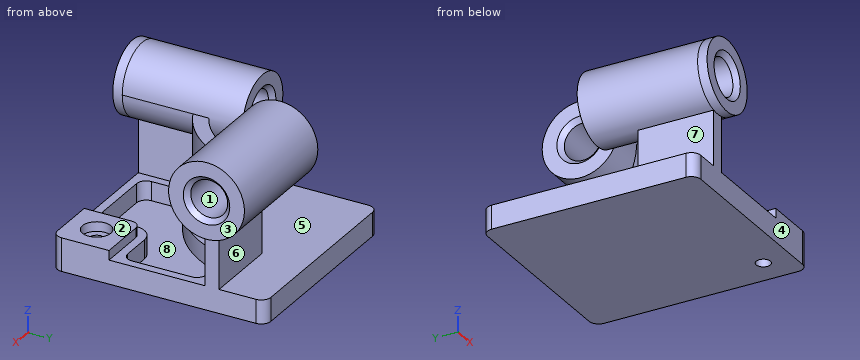
from build123d import *

# Parameters (mm, degrees)
F0_W            = 210
F0_H            = 225
F1_DEPTH        = 25
F3_DEPTH        = 95
F4_R            = 37.5
F5_DEPTH        = 10
F5_DEPTH_BACK   = 127
F6_R            = 40
F7_DEPTH        = 10
F7_DEPTH_BACK   = 127
F8_W            = 60
F8_H            = 60
F9_DEPTH        = 10
F10_R           = 10
F12_DEPTH       = 20
F14_D           = 15
F14_CBORE_D     = 30
F14_CBORE_DEPTH = 10
F15_R           = 10
F16_R           = 19.5
F17_DEPTH       = 235.001
F18_R           = 19.5
F19_DEPTH       = 220.001
F20_SIZE        = 5
F21_R           = 10


with BuildPart() as f1:
    # F0 (on Top) → F1 (new body)
    with BuildSketch(Plane.XY):
        Rectangle(F0_W, F0_H)
    extrude(amount=F1_DEPTH)

    # F2 (on face) → F3 (join)
    with BuildSketch(Plane.XY.offset(25)):
        with BuildLine():
            Line((-71, -32.5), (-71, -112.5))
            Line((-71, -112.5), (-56, -112.5))
            Line((-56, -112.5), (-56, -46.481817))
            ThreePointArc((-56, -46.481817), (7.488853, -14.988853), (38.981817, 48.5))
            Line((38.981817, 48.5), (105, 48.5))
            Line((105, 48.5), (105, 63.5))
            Line((105, 63.5), (25, 63.5))
            ThreePointArc((25, 63.5), (-3.117749, -4.382251), (-71, -32.5))
        make_face()
    extrude(amount=F3_DEPTH)

    # F4 (on face) → F5 (join, two sides)
    with BuildSketch(Plane.XZ.offset(112.5)) as f5_sk:
        with Locations((-63.5, 120)):
            Circle(F4_R)
    extrude(amount=F5_DEPTH)
    extrude(f5_sk.sketch, amount=-F5_DEPTH_BACK)

    # F6 (on face) → F7 (join, two sides)
    with BuildSketch(Plane.YZ.offset(105)) as f7_sk:
        with Locations((56, 120)):
            Circle(F6_R)
    extrude(amount=F7_DEPTH)
    extrude(f7_sk.sketch, amount=-F7_DEPTH_BACK)

    # F8 (on face) → F9 (join)
    with BuildSketch(Plane.XY.offset(25)):
        with Locations((75, -82.5)):
            Rectangle(F8_W, F8_H)
    extrude(amount=F9_DEPTH)

    # F10
    f10_edges = [f1.edges().sort_by_distance(p)[0] for p in [
        (45, -52.5, 30),
    ]]
    fillet(f10_edges, radius=F10_R)

    # F11 (on face) → F12 (cut)
    with BuildSketch(Plane.XY.offset(25)):
        with BuildLine():
            ThreePointArc((46.575508, 39.5), (13.852814, -21.352814), (-47, -54.075508))
            Line((-47, -54.075508), (-47, -103.5))
            Line((-47, -103.5), (36, -103.5))
            Line((36, -103.5), (36, -62.5))
            ThreePointArc((36, -62.5), (41.564971, -49.064971), (55, -43.5))
            Line((55, -43.5), (96, -43.5))
            Line((96, -43.5), (96, 39.5))
            Line((96, 39.5), (46.575508, 39.5))
        make_face()
    extrude(amount=-F12_DEPTH, mode=Mode.SUBTRACT)

    # F14 (through all)
    with Locations(Plane.XY.offset(35)):
        with Locations((75, -82.5)):
            CounterBoreHole(F14_D / 2, F14_CBORE_D / 2, F14_CBORE_DEPTH)

    # F15
    f15_edges = [f1.edges().sort_by_distance(p)[0] for p in [
        (-47, -54.075508, 15),
        (46.575508, 39.5, 15),
        (96, 39.5, 15),
        (96, -43.5, 15),
        (36, -103.5, 15),
        (-47, -103.5, 15),
    ]]
    fillet(f15_edges, radius=F15_R)

    # F16 (on face) → F17 (cut, through all)
    with BuildSketch(Plane.XZ.offset(122.5)):
        with Locations((-63.5, 120)):
            Circle(F16_R)
    extrude(amount=-F17_DEPTH, mode=Mode.SUBTRACT)

    # F18 (on face) → F19 (cut, through all)
    with BuildSketch(Plane.YZ.offset(115)):
        with Locations((56, 120)):
            Circle(F18_R)
    extrude(amount=-F19_DEPTH, mode=Mode.SUBTRACT)

    # F20
    f20_edges = [f1.edges().sort_by_distance(p)[0] for p in [
        (115, 36.5, 120),
        (-22, 36.5, 120),
        (-83, 14.5, 120),
        (-83, -122.5, 120),
    ]]
    chamfer(f20_edges, length=F20_SIZE)

    # F21
    f21_edges = [f1.edges().sort_by_distance(p)[0] for p in [
        (-105, -112.5, 12.5),
        (105, -112.5, 17.5),
        (105, 112.5, 12.5),
        (-105, 112.5, 12.5),
    ]]
    fillet(f21_edges, radius=F21_R)


solid = f1.part
The listing builds one solid part. Answer for the finished solid, in the listing's coordinates (mm). Face numbers are marked on the shaded views. A direction names the side the tool comes from. Coordinates: 2 decimals unless noted, no trailing zeros. Write each loop counter-clockwise with the first axis right and the second up, starting at its lowest first coordinate (ties: lowest second). Pieces come first, ordered by that corner, then holes. Notation, with made-up numbers: M 49,52 L 91,52 A21 cw 91,72 Z; hole C 76,73 d10. An arc over 180 degrees is marked long. Put each result on its own line as item: value. Start each with the question number.
1. For a pull along Z with two mould halves and no side action, classify the marked faces 1, 2 and 3 as pulls with the +Z half, pulls with the -Z half, needs draft (parallel to the pull), parting line crosses it, or undercut.
2. A cutting plane is placed at B-B on x = 75. Write down the section's boundary in (y, z), then the cut area to 3 significant figures.
3. A cutting plane is placed at A-A on y = -82.5. Write down the section's boundary in (x, z), then the cut area to 3 significant figures.
4. Consider line 1 (Y direction, x = 75, z = 19); line 2 (Z direction, x = 42.5, y = 56); line 3 (Z direction, x = -75.5, y = 10.5). Determine where each line is inside the solid, lowest interval first. Write a range as from..to.
5. A cutting plane is placed at C-C on z = 17. Write down the section's boundary in (x, y), then the cut area to 3 significant figures.
6. Flat-ended cylindrical pins translate along their axes: P1, Ø9, axis at x = 75, y = -82.5, coming from the -Z side; P2, Ø18, axis at x = 67.5, y = -69, coming from the +Z side; P3, Ø25, axis at x = -9.5, z = 38.5, coming from the -Y side; P4, Ø16, axis at y = -72, z = 17, coming from the +X side. Find the tip coordinate at first contact, or state that the pin passes through.
7. Which of the six approach directions +Z, -Z, +X, -X, +Y, -Y give full straight-line access (tool end or side, diameter ignored) to the marked faces 4, 5, 6, 7 and 8?
8. A cutting plane is placed at D-D on x = 49. Write down the section's boundary in (y, z), then the cut area to 3 significant figures.
Resolved:
1. face 1: undercut
1. face 2: pulls with the +Z half
1. face 3: needs draft
2. outline: M -112.5,0 L -90,0 L -90,25 L -97.5,25 L -97.5,35 L -112.5,35 Z; M -75,0 L 112.5,0 L 112.5,25 L 63.5,25 L 63.5,80.71 A40 ccw long 48.5,80.71 L 48.5,25 L 39.5,25 L 39.5,5 L -43.5,5 L -43.5,25 L -52.5,25 L -52.5,35 L -67.5,35 L -67.5,25 L -75,25 Z; hole C 56,120 d39
2. area: 8,550 mm2
3. outline: M -105,0 L 67.5,0 L 67.5,25 L 60,25 L 60,35 L 45,35 L 45,25 L 36,25 L 36,5 L -47,5 L -47,25 L -56,25 L -56,83.26 A37.5 ccw long -71,83.26 L -71,25 L -105,25 Z; M 82.5,0 L 105,0 L 105,35 L 90,35 L 90,25 L 82.5,25 Z; hole C -63.5,120 d39
3. area: 7,600 mm2
4. line 1: y = -112.5..-90, -75..-43.5, 39.5..112.5
4. line 2: z = 0..100.5, 139.5..160
4. line 3: z = 0..25, 84.47..103.38, 136.62..155.53
5. outline: M -105,-102.5 A10 ccw -95,-112.5 L 95,-112.5 A10 ccw 105,-102.5 L 105,102.5 A10 ccw 95,112.5 L -95,112.5 A10 ccw -105,102.5 Z; hole M -47,-93.5 A10 ccw -37,-103.5 L 26,-103.5 A10 ccw 36,-93.5 L 36,-62.5 A19 cw 55,-43.5 L 86,-43.5 A10 ccw 96,-33.5 L 96,29.5 A10 ccw 86,39.5 L 54.48,39.5 A10 ccw 44.82,32.12 A120 cw -39.62,-52.32 A10 ccw -47,-61.98 Z; hole C 75,-82.5 d15
5. area: 36,300 mm2
6. P1: passes through
6. P2: stops at z = 35
6. P3: stops at y = -36.1
6. P4: stops at x = 105
7. face 4: -Z, +X, -X, -Y
7. face 5: -X, +Y
7. face 6: +X, -X, +Y
7. face 7: -X, +Y, -Y
7. face 8: none
8. outline: M -112.5,0 L 112.5,0 L 112.5,25 L 63.5,25 L 63.5,80.71 A40 ccw long 48.5,80.71 L 48.5,25 L 37.87,25 L 37.87,5 L -44.47,5 L -44.47,25 L -54.5,25 L -54.5,35 L -112.5,35 Z; hole C 56,120 d39
8. area: 9,220 mm2
